CAD build for the part. Positions are in the model's coordinates, mm. Give positions to 0.01 mm unless a question says otherwise; leave off trailing zeros. Loops run counter-clockwise (first coordinate to the right, second up) from the corner with the lowest first, then second, coordinate; pieces in that order, holes last.
```python
from build123d import *

# Parameters (mm, degrees)
SKETCH3_R           = 23.8125
SKETCH3_R_2         = 10.3124
BOSS_EXTRUDE1_DEPTH = 1.651
FILLET1_R           = 0.1651


with BuildPart() as part:
    # Sketch3 → Boss-Extrude1 (new, symmetric)
    with BuildSketch(Plane.XY):
        with Locations(Location((0, 0, 0), (0, 0, 180))):
            Circle(SKETCH3_R)
        with Locations(Location((0, 0, 0), (0, 0, 180))):
            Circle(SKETCH3_R_2, mode=Mode.SUBTRACT)
    extrude(amount=BOSS_EXTRUDE1_DEPTH, both=True)

    # Fillet1
    fillet1_edges = [part.edges().sort_by_distance(p)[0] for p in [
        (23.8125, 0, -1.651),
        (23.8125, 0, 1.651),
        (10.3124, 0, -1.651),
        (10.3124, 0, 1.651),
    ]]
    fillet(fillet1_edges, radius=FILLET1_R)


solid = part.part
```
1. Saw through at C-C, the plane z = 0.45. List the corners of the cut face in (x, y) (1 decimal), and give its area (3 significant figures).
Responses:
outline: circle Ø47.6 at (0, 0); hole circle Ø20.6 at (0, 0)
area: 1,450 mm2
2. Saw through at A-A, the plane x = 0. List the corners of the cut face in (y, z).
Responses:
outline: (-23.81, -1.49) arc R0.17 ccw to (-23.65, -1.65) - (-10.48, -1.65) arc R0.17 ccw to (-10.31, -1.49) - (-10.31, 1.49) arc R0.17 ccw to (-10.48, 1.65) - (-23.65, 1.65) arc R0.17 ccw to (-23.81, 1.49) - close; (10.31, -1.49) arc R0.17 ccw to (10.48, -1.65) - (23.65, -1.65) arc R0.17 ccw to (23.81, -1.49) - (23.81, 1.49) arc R0.17 ccw to (23.65, 1.65) - (10.48, 1.65) arc R0.17 ccw to (10.31, 1.49) - close
3. Drop flat-ended pins along their axis: pin 1 (18.5 mm diameter, centred on x = 0, y = 0, fed in from -Z); pin 2 (1.5 mm diameter, centred on y = 9, z = 1, fed in from +X). Give the stop position or say it passes through.
Responses:
pin 1: passes through
pin 2: stops at x = 22.34
4. Probe line 1 along Y through (x, z) = (0, -0.55); line 2 along X through (y, z) = (5, 0.05); line 3 along X through (y, z) = (4.5, 0.75). List the from-to ranges inside material, lowest first.
Responses:
line 1: y = -23.81 to -10.31, 10.31 to 23.81
line 2: x = -23.28 to -9.02, 9.02 to 23.28
line 3: x = -23.38 to -9.28, 9.28 to 23.38
5. Pull direction X, two halves, no side cores. Call faces 1 (the face through (-10, 5, -1.651)), 2 (the face through (5.162, 23.246, 0.021)), 3 (the face through (7.6, -6.97, -0.02)): released by +X, released by -X, zero draft, split by the parting line, or undercut.
Responses:
face 1: zero draft
face 2: split by the parting line
face 3: undercut
